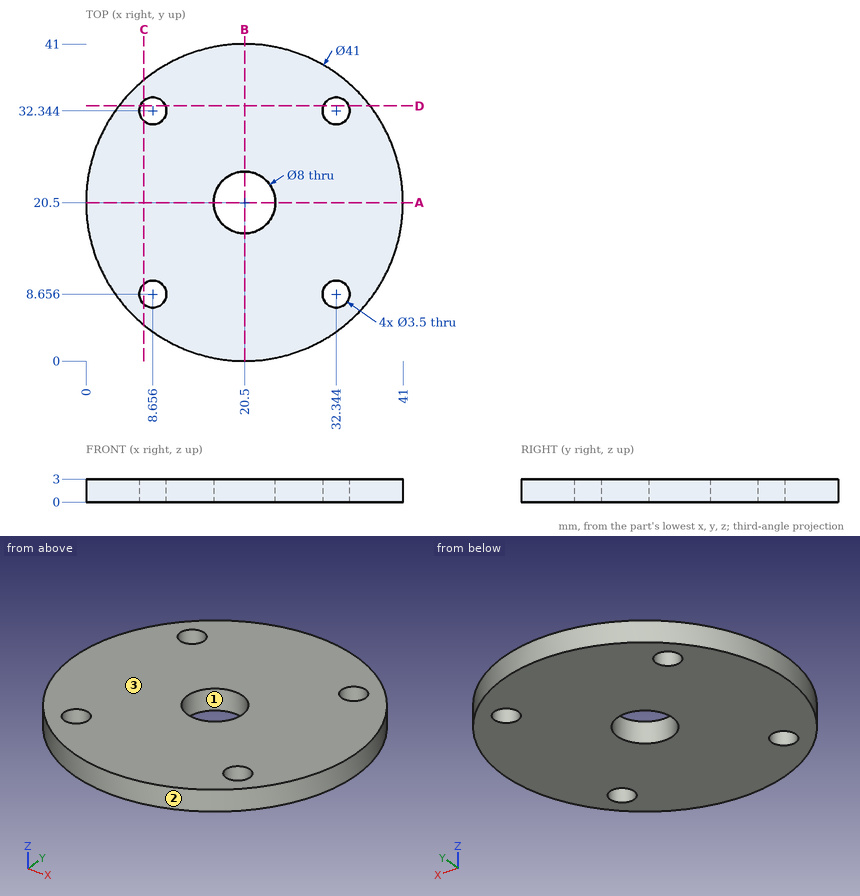
Can you work these out from the drawing? Everything is in mm from the part's minimum corner. Round coordinates to 2 decimals unless told otherwise and drop trailing zeros. Order: outer loops, then holes, each group sorted by start corner. A loop starts at its lowest first (then second) coordinate and runs counter-clockwise, first axis right, second up. Notation, with made-up numbers: (76, 43.25) -> (111, 43.25) arc R23 ccw to (111, 73.25) -> close; hole circle Ø1 at (86.25, -29.5). An arc over 180 degrees is marked (long way). Use CSV: the item, a comma, the result in double quotes.
1. I want a section at D-D on y = 33. List the corners of the cut face in (x, z) for me, and give its area (3 significant figures).
Recorded:
outline,"(4.25, 0) -> (7.03, 0) -> (7.03, 3) -> (4.25, 3) -> close; (10.28, 0) -> (30.72, 0) -> (30.72, 3) -> (10.28, 3) -> close; (33.97, 0) -> (36.75, 0) -> (36.75, 3) -> (33.97, 3) -> close"
area,"78.0 mm2"
2. I want a section at C-C on x = 7.5. List the corners of the cut face in (y, z) for me, and give its area (3 significant figures).
Recorded:
outline,"(4.65, 0) -> (7.34, 0) -> (7.34, 3) -> (4.65, 3) -> close; (9.97, 0) -> (31.03, 0) -> (31.03, 3) -> (9.97, 3) -> close; (33.66, 0) -> (36.35, 0) -> (36.35, 3) -> (33.66, 3) -> close"
area,"79.3 mm2"
3. I'm going to push a flat-ended pin straight in: P1, Ø4.5, axis at x = 32.34, y = 32.34, coming from the -Z side. Where does the tip first touch, or does it pass through?
Recorded:
P1,"stops at z = 0"
4. I want a section at A-A on y = 20.5. List the corners of the cut face in (x, z) for me, and give its area (3 significant figures).
Recorded:
outline,"(0, 0) -> (16.5, 0) -> (16.5, 3) -> (0, 3) -> close; (24.5, 0) -> (41, 0) -> (41, 3) -> (24.5, 3) -> close"
area,"99.0 mm2"
5. Thinking about a two-plate mould opening in X: for the marked faces 1, 2 and 3, which applies, pulls with the +X half, pulls with the -X half, needs draft (parallel to the pull), parting line crosses it, or undercut?
Recorded:
face 1,"undercut"
face 2,"parting line crosses it"
face 3,"needs draft"
6. I need wall thicknesses on line 1 along Y through (x, z) = (20.5, 1.85); line 2 along X through (y, z) = (33, 2.5); line 3 along X through (y, z) = (31.5, 1.5). Which ranges of each line are inside material? Lowest first, please.
Recorded:
line 1,"y = 0 to 16.5, 24.5 to 41"
line 2,"x = 4.25 to 7.03, 10.28 to 30.72, 33.97 to 36.75"
line 3,"x = 3.2 to 7.12, 10.19 to 30.81, 33.88 to 37.8"
